from build123d import *

# Parameters (mm, degrees)
F0_W      = 98.425
F0_H      = 53.975
F1_DEPTH  = 8.89
F3_DEPTH  = 9.525
F5_DEPTH  = 19.05
F7_DEPTH  = 7.9248
F8_W      = 9.525
F8_H      = 53.975
F9_DEPTH  = 9.525
F10_W     = 9.525
F10_H     = 38.1
F11_DEPTH = 7.9248
F12_R     = 3.041543
F13_DEPTH = 25.4
F14_W     = 9.525
F14_H     = 9.525
F15_DEPTH = 26.9748


with BuildPart() as f1:
    # F0 (on Top) → F1 (new body)
    with BuildSketch(Plane.XY):
        with Locations((49.2125, 26.9875)):
            Rectangle(F0_W, F0_H)
    extrude(amount=F1_DEPTH)

    # F2 (on face) → F3 (join)
    with BuildSketch(Plane.XY.offset(8.89)):
        Polygon((25.4, 0), (34.925, 0), (34.925, 38.1), (44.45, 38.1), (44.45, 53.975), (25.4, 53.975), align=None)
    extrude(amount=F3_DEPTH)

    # F4 (on face) → F5 (join)
    with BuildSketch(Plane.XY.offset(8.89)):
        Polygon((73.025, 53.975), (63.5, 53.975), (63.5, 38.1), (48.8696, 3.41884), (48.8696, 0), (56.952347, 0), (73.025, 38.1), align=None)
    extrude(amount=F5_DEPTH)

    # F6 (on face) → F7 (join)
    with BuildSketch(Plane.XY.offset(27.94)):
        Polygon((48.8696, 0), (56.952347, 0), (73.025, 38.1), (63.5, 38.1), (48.8696, 3.41884), align=None)
    extrude(amount=F7_DEPTH)

    # F8 (on face) → F9 (join)
    with BuildSketch(Plane.XY.offset(18.415)):
        with Locations((30.1625, 26.9875)):
            Rectangle(F8_W, F8_H)
    extrude(amount=F9_DEPTH)

    # F10 (on face) → F11 (join)
    with BuildSketch(Plane.XY.offset(27.94)):
        with Locations((30.1625, 19.05)):
            Rectangle(F10_W, F10_H)
    extrude(amount=F11_DEPTH)

    # F12 (on face) → F13 (cut)
    with BuildSketch(Plane.XY.offset(8.89)):
        with Locations((6.35, 47.625)):
            Circle(F12_R)
        with Locations((6.35, 6.35)):
            Circle(F12_R)
        with Locations((92.075, 6.35)):
            Circle(F12_R)
        with Locations((92.075, 47.625)):
            Circle(F12_R)
    extrude(amount=-F13_DEPTH, mode=Mode.SUBTRACT)

    # F14 (on face) → F15 (cut, through all)
    with BuildSketch(Plane.XY.offset(35.8648)):
        with Locations((30.1625, 4.7625)):
            Rectangle(F14_W, F14_H)
    extrude(amount=-F15_DEPTH, mode=Mode.SUBTRACT)


solid = f1.part
Here's how the part is built. I have some questions about the finished solid (model axes, mm). A direction names the side the tool comes from. Give positions to 0.01 mm unless a question says otherwise; leave off trailing zeros. Loops run counter-clockwise (first coordinate to the right, second up) from the corner with the lowest first, then second, coordinate; pieces in that order, holes last. Notation, with made-up numbers: (-32.5, 68.25) -> (26.5, 68.25) arc R24 ccw to (26.5, 92.25) -> close; hole circle Ø3 at (18.25, -25.5). An arc over 180 degrees is marked (long way). Answer as a JSON object with one key per item and string values. Group by question number.
Item 1: Will these pins go through, and if not, where does the flat tip stop? pin 1 (17.5 mm diameter, centred on y = 49, z = 22, fed in from -X); pin 2 (3.5 mm diameter, centred on x = 92.075, y = 6.35, fed in from +Z); pin 3 (8.5 mm diameter, centred on x = 28.5, z = 33.5, fed in from +Y); pin 4 (4 mm diameter, centred on y = 1, z = 23.5, fed in from -X).
Item 2: Imagine slicing it at B-B on z = 33.5. Write out the boundary of the cut face in (x, y) (3 decimals).
Item 3: I need wall thicknesses on L1, parallel to Y at x = 6, z = 5 (3 decimals); L2, parallel to X at y = 6, z = 5 (3 decimals); L3, parallel to X at y = 47, z = 11 (3 decimals). Which ranges of each line are inside material? Lowest first, please.
Item 4: Imagine slicing it at A-A on x = 6.35. Write out the boundary of the cut face in (y, z) (3 decimals), then the cut area to 3 significant figures.
Item 5: On a 3-axis mill with a long thin cutter (end or side, diameter ignored), from which of +Z, -Z, +X, -X, +Y, -Y can I reach the whole of each face in a straight line? I mean faces 1 (the flat face through (82, 21, 8.89)), 2 (the flat face through (73.025, 46, 18)), 3 (the flat face through (68, 46, 27.94)). Say none if no direction works.
Item 6: Thinking about a two-plate mould opening in X: for faces 4 (the flat face through (63.5, 46, 18)), 5 (the flat face through (98.425, 27, 4)), 6 (the flat face through (30, 9.525, 23)), which applies, pulls with the +X half, pulls with the -X half, needs draft (parallel to the pull), parting line crosses it, or undercut?
Item 7: Imagine slicing it at D-D on z = 12.5. Write out the boundary of the cut face in (x, y) (3 decimals), then the cut area to 3 significant figures.
Item 8: Imagine slicing it at C-C on y = 6.35. Write out the boundary of the cut face in (x, z) (3 decimals).
Answer list:
{
 "1": {"pin 1": "stops at x = 25.4", "pin 2": "passes through", "pin 3": "stops at y = 38.1", "pin 4": "stops at x = 48.87"},
 "2": {"outline": "(25.4, 9.525) -> (34.925, 9.525) -> (34.925, 38.1) -> (25.4, 38.1) -> close; (48.87, 0) -> (56.952, 0) -> (73.025, 38.1) -> (63.5, 38.1) -> (48.87, 3.419) -> close"},
 "3": {"L1": "y = 0 to 3.329, 9.371 to 44.604, 50.646 to 53.975", "L2": "x = 0 to 3.329, 9.371 to 89.054, 95.096 to 98.425", "L3": "x = 25.4 to 44.45, 63.5 to 73.025"},
 "4": {"outline": "(0, 0) -> (3.308, 0) -> (3.308, 8.89) -> (0, 8.89) -> close; (9.392, 0) -> (44.583, 0) -> (44.583, 8.89) -> (9.392, 8.89) -> close; (50.667, 0) -> (53.975, 0) -> (53.975, 8.89) -> (50.667, 8.89) -> close", "area": "372 mm2"},
 "5": {"face 1": "+Z, +X, -Y", "face 2": "+Z, +X, +Y, -Y", "face 3": "+Z, +X, -X, +Y"},
 "6": {"face 4": "undercut", "face 5": "pulls with the +X half", "face 6": "needs draft"},
 "7": {"outline": "(25.4, 9.525) -> (34.925, 9.525) -> (34.925, 38.1) -> (44.45, 38.1) -> (44.45, 53.975) -> (25.4, 53.975) -> close; (48.87, 0) -> (56.952, 0) -> (73.025, 38.1) -> (73.025, 53.975) -> (63.5, 53.975) -> (63.5, 38.1) -> (48.87, 3.419) -> close", "area": "1,090 mm2"},
 "8": {"outline": "(0, 0) -> (3.308, 0) -> (3.308, 8.89) -> (0, 8.89) -> close; (9.392, 0) -> (89.033, 0) -> (89.033, 8.89) -> (59.631, 8.89) -> (59.631, 35.865) -> (50.106, 35.865) -> (50.106, 8.89) -> (9.392, 8.89) -> close; (95.117, 0) -> (98.425, 0) -> (98.425, 8.89) -> (95.117, 8.89) -> close"}
}
